The figure shows three views and two pictorial views of one solid part (mm, origin at its lowest corner). Answer the questions. A direction names the side the tool comes from. Round coordinates to 2 decimals unless told otherwise and drop trailing zeros. Order: outer loops, then holes, each group sorted by start corner. A loop starts at its lowest first (then second) coordinate and runs counter-clockwise, first axis right, second up. Notation, with made-up numbers: M -0.5,63.5 L 10.5,63.5 A18 ccw 10.5,92.5 Z; hole C 21,-37.75 d8. An arc over 180 degrees is marked long. Answer as CSV lines item,"result".
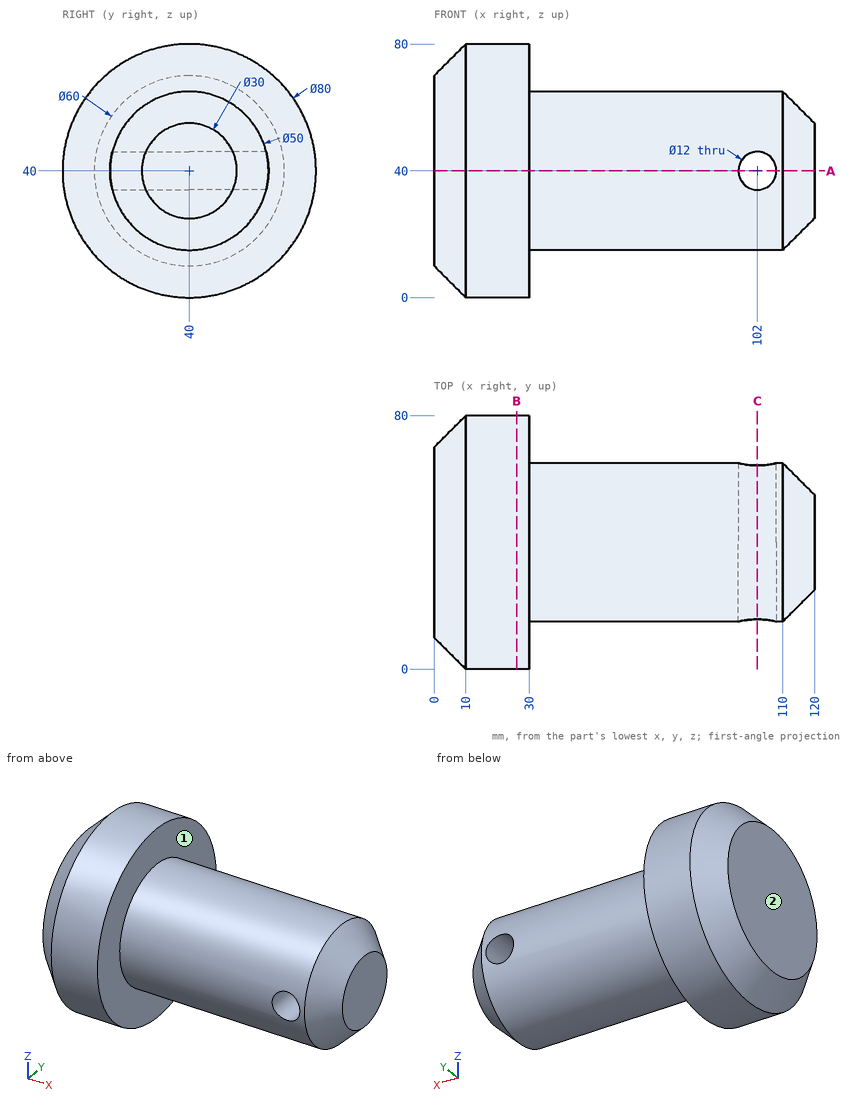
Item 1: A cutting plane is placed at B-B, the plane x = 26. Determine the outline of the cut face in (y, z).
Ans:
outline,"C 40,40 d80"
Item 2: Flat-ended cylindrical pins translate along their axes: pin 1 (14 mm diameter, centred on x = 102, z = 40, fed in from -Y); pin 2 (12 mm diameter, centred on x = 90.5, y = 21.5, fed in from +Z); pin 3 (12 mm diameter, centred on x = 16, z = 24.5, fed in from +Y); pin 4 (2 mm diameter, centred on y = 33.5, z = 44.5, fed in from -X). Find the tip coordinate at first contact, or state that the pin passes through.
Ans:
pin 1,"y = 15"
pin 2,"z = 61.65"
pin 3,"y = 78.86"
pin 4,"x = 0"
Item 3: Find the intervals of material crossed by probe 1 along X at (y, z) = (21.5, 40); probe 2 along Z at (x, y) = (62, 41); probe 3 along Z at (x, y) = (103.5, 23.5), in increasing order. Write a range as [from, to].
Ans:
probe 1,"[0, 96], [108, 116.5]"
probe 2,"[15.02, 64.98]"
probe 3,"[21.22, 34.19], [45.81, 58.78]"
Item 4: A cutting plane is placed at A-A, the plane z = 40. Determine the outline of the cut face in (x, y), and give its area (3 significant figures).
Ans:
outline,"M 0,10 L 10,0 L 30,0 L 30,15 L 96,15 L 96,65 L 30,65 L 30,80 L 10,80 L 0,70 Z; M 108,15 L 110,15 L 120,25 L 120,55 L 110,65 L 108,65 Z"
area,"6,100 mm2"
Item 5: A cutting plane is placed at C-C, the plane x = 102. Determine the outline of the cut face in (y, z).
Ans:
outline,"M 15.73,34 A25 ccw 64.27,34 Z; M 15.73,46 L 64.27,46 A25 ccw Z"
Item 6: A tool of negligible diameter and unlimited length cuts with its end or side. For the marked faces 1 and 2, from which of +Z, -Z, +X, -X, +Y, -Y can it reach the whole face along a straight path? Write none if from no direction.
Ans:
face 1,"+X"
face 2,"+Z, -Z, -X, +Y, -Y"
